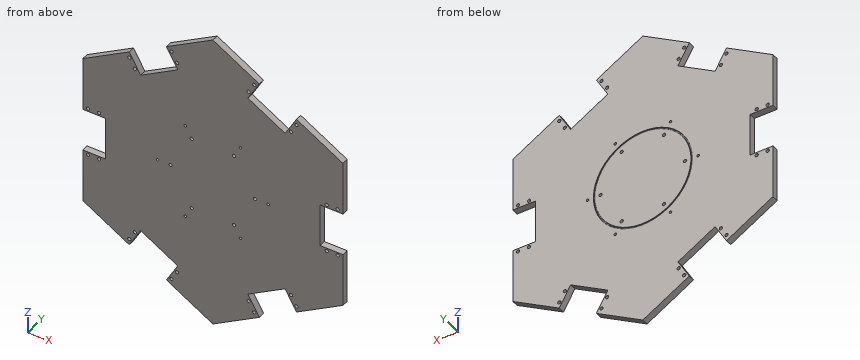
```python
from build123d import *

# Parameters (mm, degrees)
BOSS_EXTRUDE1_DEPTH     = 10
CUT_EXTRUDE1_DEPTH      = 306.668665933
CUT_EXTRUDE1_DEPTH_BACK = 306.668665933
SKETCH2_R               = 2.5
SKETCH2_W               = 35
SKETCH2_H               = 66
FILLET1_R               = 0.254
CUT_EXTRUDE2_DEPTH      = 306.668665933
CUT_EXTRUDE2_DEPTH_BACK = 306.668665933
SKETCH5_R               = 2
SKETCH5_R_2             = 2.5


with BuildPart() as part:
    # Sketch1 → Boss-Extrude1 (new body)
    with BuildSketch(Plane(origin=(0, 0, 0), x_dir=(1, 0, 0), z_dir=(0, 1, 0))):
        Polygon((-200, 115.470053838), (0, 230.940107676), (200, 115.470053838), (200, -115.470053838), (0, -230.940107676), (-200, -115.470053838), align=None)
    extrude(amount=BOSS_EXTRUDE1_DEPTH)

    # Sketch2 → Cut-Extrude1 (cut, two sides: drawn at the far end of the back side and taken through both)
    with BuildSketch(Plane(origin=(0, 10, 0), x_dir=(1, 0, 0), z_dir=(0, 1, 0)).offset(-CUT_EXTRUDE1_DEPTH_BACK)):
        with Locations(Location((175, 37.5, 0), (0, 0, 270))):
            Circle(SKETCH2_R)
        with Locations((182.5, 0)):
            Rectangle(SKETCH2_W, SKETCH2_H)
        with Locations(Location((175, -37.5, 0), (0, 0, 270))):
            Circle(SKETCH2_R)
        Polygon((71.421161675, -189.705080757), (128.578838325, -156.705080757), (111.078838325, -126.394191624), (53.921161675, -159.394191624), align=None)
        Polygon((111.078838325, 126.394191624), (128.578838325, 156.705080757), (71.421161675, 189.705080757), (53.921161675, 159.394191624), align=None)
        Polygon((-128.578838325, -156.705080757), (-71.421161675, -189.705080757), (-53.921161675, -159.394191624), (-111.078838325, -126.394191624), align=None)
        Polygon((-53.921161675, 159.394191624), (-71.421161675, 189.705080757), (-128.578838325, 156.705080757), (-111.078838325, 126.394191624), align=None)
        with Locations((-182.5, 0)):
            Rectangle(SKETCH2_W, SKETCH2_H)
        with Locations(Location((192, 37.5, 0), (0, 0, 270))):
            Circle(SKETCH2_R)
        with Locations(Location((192, -37.5, 0), (0, 0, 270))):
            Circle(SKETCH2_R)
        with Locations(Location((119.975952642, -132.804445662, 0), (0, 0, 270))):
            Circle(SKETCH2_R)
        with Locations(Location((128.475952642, -147.526877527, 0), (0, 0, 270))):
            Circle(SKETCH2_R)
        with Locations(Location((55.024047358, -170.304445662, 0), (0, 0, 270))):
            Circle(SKETCH2_R)
        with Locations(Location((63.524047358, -185.026877527, 0), (0, 0, 270))):
            Circle(SKETCH2_R)
        with Locations(Location((-55.024047358, -170.304445662, 0), (0, 0, 270))):
            Circle(SKETCH2_R)
        with Locations(Location((-63.524047358, -185.026877527, 0), (0, 0, 270))):
            Circle(SKETCH2_R)
        with Locations(Location((-119.975952642, -132.804445662, 0), (0, 0, 270))):
            Circle(SKETCH2_R)
        with Locations(Location((-128.475952642, -147.526877527, 0), (0, 0, 270))):
            Circle(SKETCH2_R)
        with Locations(Location((-175, -37.5, 0), (0, 0, 270))):
            Circle(SKETCH2_R)
        with Locations(Location((-192, -37.5, 0), (0, 0, 270))):
            Circle(SKETCH2_R)
        with Locations(Location((-175, 37.5, 0), (0, 0, 270))):
            Circle(SKETCH2_R)
        with Locations(Location((-192, 37.5, 0), (0, 0, 270))):
            Circle(SKETCH2_R)
        with Locations(Location((-119.975952642, 132.804445662, 0), (0, 0, 270))):
            Circle(SKETCH2_R)
        with Locations(Location((-128.475952642, 147.526877527, 0), (0, 0, 270))):
            Circle(SKETCH2_R)
        with Locations(Location((-55.024047358, 170.304445662, 0), (0, 0, 270))):
            Circle(SKETCH2_R)
        with Locations(Location((-63.524047358, 185.026877527, 0), (0, 0, 270))):
            Circle(SKETCH2_R)
        with Locations(Location((55.024047358, 170.304445662, 0), (0, 0, 270))):
            Circle(SKETCH2_R)
        with Locations(Location((63.524047358, 185.026877527, 0), (0, 0, 270))):
            Circle(SKETCH2_R)
        with Locations(Location((119.975952642, 132.804445662, 0), (0, 0, 270))):
            Circle(SKETCH2_R)
        with Locations(Location((128.475952642, 147.526877527, 0), (0, 0, 270))):
            Circle(SKETCH2_R)
    extrude(amount=CUT_EXTRUDE1_DEPTH + CUT_EXTRUDE1_DEPTH_BACK, mode=Mode.SUBTRACT)

    # Cut-Sweep1: sweep along a path in Sketch4
    with BuildLine(Plane(origin=(0, 10, 0), x_dir=(1, 0, 0), z_dir=(0, 1, 0))) as cut_sweep1_path:
        CenterArc((0, 0), 75, 0, 360)
    # Sketch3 → Cut-Sweep1 (sweep, cut)
    with BuildSketch(Plane.XY):
        with BuildLine():
            Line((74.11, 10), (74.11, 8.984))
            ThreePointArc((74.11, 8.984), (74.184394878, 8.804394878), (74.364, 8.73))
            Line((74.364, 8.73), (75.636, 8.73))
            ThreePointArc((75.636, 8.73), (75.815605122, 8.804394878), (75.89, 8.984))
            Line((75.89, 8.984), (75.89, 10))
            Line((75.89, 10), (74.11, 10))
        make_face()
    sweep(path=cut_sweep1_path.line, mode=Mode.SUBTRACT)

    # Fillet1
    fillet1_edges = [part.edges().sort_by_distance(p)[0] for p in [
        (-75.89, 10, 0),
        (-74.11, 10, 0),
    ]]
    fillet(fillet1_edges, radius=FILLET1_R)

    # Sketch5 → Cut-Extrude2 (cut, two sides: drawn at the far end of the back side and taken through both)
    with BuildSketch(Plane(origin=(0, 10, 0), x_dir=(1, 0, 0), z_dir=(0, 1, 0)).offset(-CUT_EXTRUDE2_DEPTH_BACK)):
        with Locations(Location((85, 0, 0), (0, 0, 270))):
            Circle(SKETCH5_R)
        with Locations(Location((42.5, -73.612159322, 0), (0, 0, 270))):
            Circle(SKETCH5_R)
        with Locations(Location((-42.5, -73.612159322, 0), (0, 0, 270))):
            Circle(SKETCH5_R)
        with Locations(Location((-85, 0, 0), (0, 0, 270))):
            Circle(SKETCH5_R)
        with Locations(Location((-42.5, 73.612159322, 0), (0, 0, 270))):
            Circle(SKETCH5_R)
        with Locations(Location((42.5, 73.612159322, 0), (0, 0, 270))):
            Circle(SKETCH5_R)
        with Locations(Location((65, 0, 0), (0, 0, 270))):
            Circle(SKETCH5_R_2)
        with Locations(Location((32.5, -56.291651246, 0), (0, 0, 270))):
            Circle(SKETCH5_R_2)
        with Locations(Location((-32.5, -56.291651246, 0), (0, 0, 270))):
            Circle(SKETCH5_R_2)
        with Locations(Location((-65, 0, 0), (0, 0, 270))):
            Circle(SKETCH5_R_2)
        with Locations(Location((-32.5, 56.291651246, 0), (0, 0, 270))):
            Circle(SKETCH5_R_2)
        with Locations(Location((32.5, 56.291651246, 0), (0, 0, 270))):
            Circle(SKETCH5_R_2)
    extrude(amount=CUT_EXTRUDE2_DEPTH + CUT_EXTRUDE2_DEPTH_BACK, mode=Mode.SUBTRACT)


solid = part.part
```
The listing builds one solid part. Answer for the finished solid, in the listing's coordinates (mm). Coordinates: 2 decimals unless noted, no trailing zeros.
Q1. Find the intervals of material crossed by line 1 along X through (y, z) = (3.25, 37.5); line 2 along X through (y, z) = (6.25, 0); line 3 along Z through (x, y) = (192, 4), in increasing order.
Returned:
line 1: x = -200 to -194.5, -189.5 to -177.5, -172.5 to 172.5, 177.5 to 189.5, 194.5 to 200
line 2: x = -165 to -87, -83 to -67.5, -62.5 to 62.5, 67.5 to 83, 87 to 165
line 3: z = -120.09 to -40, -35 to -33, 33 to 35, 40 to 120.09
Q2. Section A-A, the plane y = 1.75 is taken. Give the number of separate pieces and of enclosed holes in the cut face, then the cut area to 3 significant figures.
Returned:
separate pieces: 1
enclosed holes: 36
area: 124,000 mm2
Q3. Given P1, Ø2.5, axis at x = -85, z = 0, coming from the +Y side; P2, Ø3, axis at y = 4, z = 4.5, coming from the -X side, each flat-ended and moving along its own axis, determine where each tip first touches the part or whether it passes through.
Returned:
P1: passes through
P2: stops at x = -165
